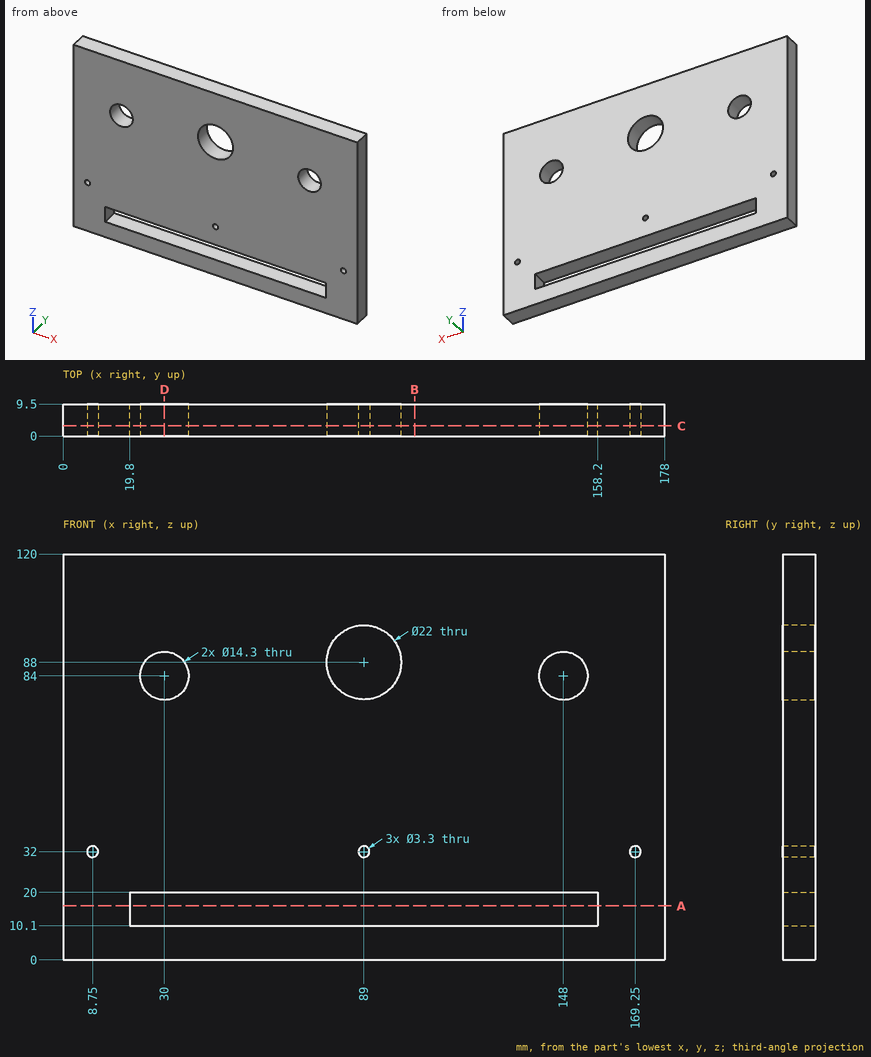
Geometry check sheet. Reference: drawing and pictorial views, mm from the part's lowest x, y, z. Give positions to 0.01 mm unless a question says otherwise; leave off trailing zeros. Order: outer loops, then holes, each group sorted by start corner. A loop starts at its lowest first (then second) coordinate and runs counter-clockwise, first axis right, second up. Notation, with made-up numbers: (-15.75, 59) - (15.25, 59) arc R31 ccw to (15.25, 90) - close; hole circle Ø9 at (40, 65.25). An arc over 180 degrees is marked (long way). Answer as CSV lines item,"result".
1. Section check B-B (x = 104). Record the boundary of the cut face in (y, z).
Result sheet:
outline,"(0, 0) - (9.5, 0) - (9.5, 10.1) - (0, 10.1) - close; (0, 20) - (9.5, 20) - (9.5, 120) - (0, 120) - close"
2. Scan lines: probe 1 along Z at (x, y) = (30, 5); probe 2 along Z at (x, y) = (89, 3.25); probe 3 along X at (y, z) = (5, 32). Record each from-to range of solid material in increasing order. Write a range as from..to.
Result sheet:
probe 1,"0..10.1, 20..76.85, 91.15..120"
probe 2,"0..10.1, 20..30.35, 33.65..77, 99..120"
probe 3,"0..7.1, 10.4..87.35, 90.65..167.6, 170.9..178"
3. Go/stop test with a flat-tipped pin: P1, Ø8.5, axis at x = 148, z = 84, coming from the +Y side. Record where the tip stops, or that it passes through.
Result sheet:
P1,"through"
4. Section check A-A (z = 16). Record the boundary of the cut face in (x, y).
Result sheet:
outline,"(0, 0) - (19.8, 0) - (19.8, 9.5) - (0, 9.5) - close; (158.2, 0) - (178, 0) - (178, 9.5) - (158.2, 9.5) - close"
5. Section check C-C (y = 3). Record the boundary of the cut face in (x, z), then the cut area to 3 significant figures.
Result sheet:
outline,"(0, 0) - (178, 0) - (178, 120) - (0, 120) - close; hole circle Ø3.3 at (8.75, 32); hole (19.8, 10.1) - (158.2, 10.1) - (158.2, 20) - (19.8, 20) - close; hole circle Ø14.3 at (30, 84); hole circle Ø22 at (89, 88); hole circle Ø3.3 at (89, 32); hole circle Ø14.3 at (148, 84); hole circle Ø3.3 at (169.25, 32)"
area,"19,300 mm²"
6. Section check D-D (x = 30). Record the boundary of the cut face in (y, z), then the cut area to 3 significant figures.
Result sheet:
outline,"(0, 0) - (9.5, 0) - (9.5, 10.1) - (0, 10.1) - close; (0, 20) - (9.5, 20) - (9.5, 76.85) - (0, 76.85) - close; (0, 91.15) - (9.5, 91.15) - (9.5, 120) - (0, 120) - close"
area,"910 mm²"
